```python
from build123d import *

# Parameters (mm, degrees)
EXTRUDE_2_DEPTH      = 16
SKETCH_31_W          = 4.8
SKETCH_31_H          = 46.486909283
CUT_EXTRUDE_6_DEPTH  = 67.474283586
SKETCH_32_W          = 4.8
SKETCH_32_H          = 14.308405558
CUT_EXTRUDE_7_DEPTH  = 16
FILLET_1_R           = 10
FILLET_2_R           = 10
SKETCH_39_W          = 1.7
SKETCH_39_H          = 35
EXTRUDE_1_DEPTH      = 1
SKETCH_40_W          = 1
SKETCH_40_H          = 4.8
CUT_EXTRUDE_8_DEPTH  = 10
SKETCH_41_W          = 3.264842031
SKETCH_41_H          = 6.457557915
CUT_EXTRUDE_9_DEPTH  = 10
SKETCH_42_W          = 4.8
SKETCH_42_H          = 1.68
CUT_EXTRUDE_10_DEPTH = 10
EXTRUDE_3_DEPTH      = 16


with BuildPart() as part:
    # 草图28 → 拉伸-薄壁2 (new body)
    with BuildSketch(Plane.XY):
        Polygon((0, 0), (0, 18), (1.217228096, 64.484065611), (2.216885421, 64.457888663), (1, 17.986909283), (1, 0), align=None)
    extrude(amount=EXTRUDE_2_DEPTH)

    # 草图31 → 切除-拉伸6 (cut, through all)
    with BuildSketch(Plane(origin=(0.528633719, -0.013842761, 0), x_dir=(0, 0, -1), z_dir=(0.9996573249755574, -0.02617694830787331, 0))):
        with Locations((-13.6, 41.250377209)):
            Rectangle(SKETCH_31_W, SKETCH_31_H)
        with Locations((-2.4, 41.250377209)):
            Rectangle(SKETCH_31_W, SKETCH_31_H)
    extrude(amount=-CUT_EXTRUDE_6_DEPTH, mode=Mode.SUBTRACT)

    # 草图32 → 切除-拉伸7 (cut)
    with BuildSketch(Plane(origin=(1, 0, 0), x_dir=(0, 0, -1), z_dir=(1, 0, 0))):
        with Locations((-13.6, 10.832706504)):
            Rectangle(SKETCH_32_W, SKETCH_32_H)
        with Locations((-2.4, 10.832706504)):
            Rectangle(SKETCH_32_W, SKETCH_32_H)
    extrude(amount=-CUT_EXTRUDE_7_DEPTH, mode=Mode.SUBTRACT)

    # 圆角1
    # the kernel refuses this fillet: 10 mm, written as the material it takes off along each edge
    with BuildSketch(Plane(origin=(0, 18, -0.327267927), x_dir=(0, -1, 0), z_dir=(0, 0, 1))) as fillet_1_piece_1:
        with BuildLine():
            CenterArc((FILLET_1_R * 0.0130907170848, FILLET_1_R), FILLET_1_R, 268.5, 1.5)
            Line((-FILLET_1_R * 0.013086231223, FILLET_1_R * 0.000342675024443), (0, 0))
            Line((0, 0), (FILLET_1_R * 0.0130907170848, 0))
        make_face()
    extrude(amount=16.654535854, mode=Mode.SUBTRACT)

    # 圆角2
    # the kernel refuses this fillet: 10 mm, written as the material it adds along each edge
    with BuildSketch(Plane(origin=(1, 17.986909283, 4.8), x_dir=(0, -1, 0), z_dir=(0, 0, 1))) as fillet_2_piece_1:
        with BuildLine():
            CenterArc((FILLET_2_R * 0.0130907170848, FILLET_2_R), FILLET_2_R, 268.5, 1.5)
            Line((-FILLET_2_R * 0.013086231223, FILLET_2_R * 0.000342675024443), (0, 0))
            Line((0, 0), (FILLET_2_R * 0.0130907170848, 0))
        make_face()
    extrude(amount=6.4)

    # 草图39 → 凸台-拉伸1 (add)
    with BuildSketch(Plane(origin=(-0.471023606, 0.012334187, 0), x_dir=(0, 0, 1), z_dir=(-0.9996573249755574, 0.026176948307873305, 0))):
        with Locations((12.05, 46.99383185)):
            Rectangle(SKETCH_39_W, SKETCH_39_H)
        with Locations((3.95, 46.99383185)):
            Rectangle(SKETCH_39_W, SKETCH_39_H)
    extrude(amount=-EXTRUDE_1_DEPTH)

    # 草图40 → 切除-拉伸8 (cut)
    with BuildSketch(Plane(origin=(0.471366281, 18.000752044, 0), x_dir=(0.9996573249755574, -0.02617694830787331, 0), z_dir=(0.02617694830787331, 0.9996573249755574, 0))):
        with Locations((0.02881493, -13.6)):
            Rectangle(SKETCH_40_W, SKETCH_40_H)
    extrude(amount=-CUT_EXTRUDE_8_DEPTH, mode=Mode.SUBTRACT)

    # 草图41 → 切除-拉伸9 (cut)
    with BuildSketch(Plane(origin=(0.471366281, 18.000752044, 0), x_dir=(0.9996573249755574, -0.02617694830787331, 0), z_dir=(0.02617694830787331, 0.9996573249755574, 0))):
        with Locations((-1.103606086, -1.571221043)):
            Rectangle(SKETCH_41_W, SKETCH_41_H)
    extrude(amount=-CUT_EXTRUDE_9_DEPTH, mode=Mode.SUBTRACT)

    # 草图42 → 切除-拉伸10 (cut)
    with BuildSketch(Plane(origin=(1, 0, 0), x_dir=(0, 0, -1), z_dir=(1, 0, 0))):
        with Locations((-2.4, 2.838503725)):
            Rectangle(SKETCH_42_W, SKETCH_42_H)
        with Locations((-13.6, 2.838503725)):
            Rectangle(SKETCH_42_W, SKETCH_42_H)
    extrude(amount=-CUT_EXTRUDE_10_DEPTH, mode=Mode.SUBTRACT)

    # 草图44 → 拉伸-薄壁3 (add)
    with BuildSketch(Plane(origin=(0, 0, 0), x_dir=(-1, 0, 0), z_dir=(0, 0, -1))):
        Polygon((0, 0), (0, -8), (1.710100717, -12.698463104), (0.770408096, -13.040483247), (-1, -8.176326981), (-1, 0), align=None)
    extrude(amount=-EXTRUDE_3_DEPTH)


solid = part.part
```
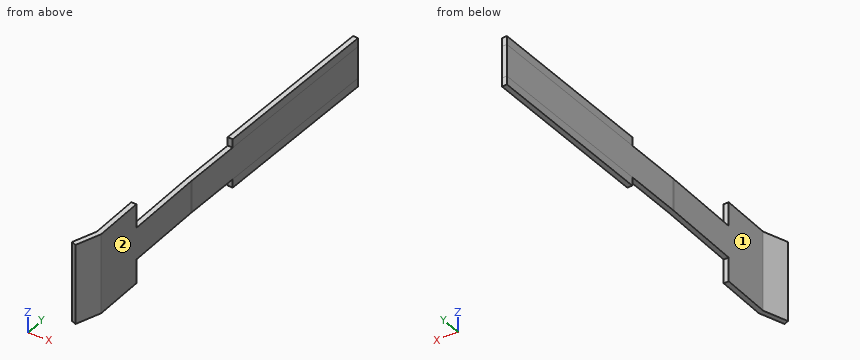
Geometry check sheet. Reference: the model listing, model coordinates, mm. Face numbers are marked on the shaded views. A direction names the side the tool comes from. Coordinates: 2 decimals unless noted, no trailing zeros. Order: outer loops, then holes, each group sorted by start corner. A loop starts at its lowest first (then second) coordinate and runs counter-clockwise, first axis right, second up. Notation, with made-up numbers: M 34.25,-33.75 L 66.25,-33.75 A31 cw 66.25,5.25 Z; hole C 30.25,41 d4. An arc over 180 degrees is marked long. One line per question, with ' | ' between items. Start each with the question number.
Item 1: Gauge pin test, flat ends, axial feed: pin 1 (2 mm diameter, centred on x = 0.5, y = 9.5, fed in from +Z); pin 2 (8 mm diameter, centred on y = 0, z = 5, fed in from -X); pin 3 (1 mm diameter, centred on x = 1.5, y = 45.5, fed in from -Z). Record the tip position at first contact, or that the pin passes through.
Item 2: Cross-section at C-C on z = 7. Enter the section's corners in (x, y), then the cut area to 3 significant figures.
Item 3: Set-up check for the marked faces 1 and 2: record each of +Z, -Z, +X, -X, +Y, -Y from which the full face is reachable in a straight line by a thin tool's end or side.
Item 4: Cross-section at D-D on y = 39. Enter the section's corners in (x, z).
Item 5: Cross-section at B-B on y = 4.5. Enter the section's corners in (x, z), then the cut area to 3 significant figures.
Item 6: Cross-section at A-A on z = 14.25. Enter the section's corners in (x, y), then the cut area to 3 significant figures.
Item 7: Material ranges on L1, parallel to X at y = 10.5, z = 8; L2, parallel to Z at x = 0.85, y = 26.5; L3, parallel to Z at x = 1.3, y = 36, recorded low to high. Write a range as [from, to].
Findings:
1) pin 1: stops at z = 11.2 | pin 2: stops at x = 0 | pin 3: stops at z = 3.1
2) outline: M -1.71,-12.7 L -0.77,-13.04 L 1,-8.18 L 1,17.86 A10 cw 1,18.12 L 2.22,64.46 L 1.22,64.48 L 0,18.13 A10 ccw 0,17.87 L 0,-8 Z | area: 77.7 mm²
3) face 1: +Z, -Z, -X, +Y | face 2: +Z, -Z, +X, -Y
4) outline: M 0.55,3.1 L 1.55,3.1 L 1.55,12.9 L 0.55,12.9 Z
5) outline: M 0,4.8 L 1,4.8 L 1,11.2 L 0,11.2 Z | area: 6.40 mm²
6) outline: M -1.71,-12.7 L -0.77,-13.04 L 1,-8.18 L 1,2 L 0,2 L 0,-8 Z | area: 15.2 mm²
7) L1: x = [0, 1] | L2: z = [4.8, 11.2] | L3: z = [3.1, 12.9]
